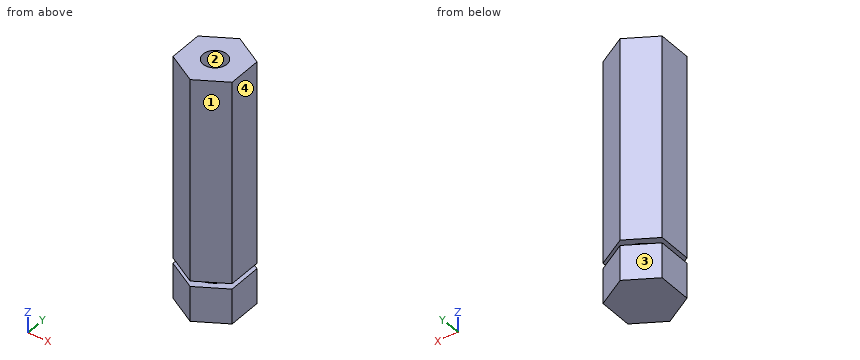
from build123d import *

# Parameters (mm, degrees)
BOSS_EXTRUDE1_DEPTH         = 26.19375
F_1_4_20_TAPPED_HOLE1_D     = 5.1054
F_1_4_20_TAPPED_HOLE1_DEPTH = 19.05
F_1_4_20_TAPPED_HOLE1_TIP   = 1.533816902
SKETCH5_W                   = 1.1684
SKETCH5_H                   = 4.843148419


with BuildPart() as part:
    # Sketch1 → Boss-Extrude1 (new body, symmetric)
    with BuildSketch(Plane.XY):
        Polygon((-6.35, 3.666174209), (-6.35, -3.666174209), (0, -7.332348419), (6.35, -3.666174209), (6.35, 3.666174209), (0, 7.332348419), align=None)
    extrude(amount=BOSS_EXTRUDE1_DEPTH, both=True)

    # 1/4-20 Tapped Hole1
    with Locations(Plane.XY.offset(26.19375)):
        with Locations((0, 0)):
            Hole(F_1_4_20_TAPPED_HOLE1_D / 2, depth=F_1_4_20_TAPPED_HOLE1_DEPTH)
            with Locations((0, 0, -(F_1_4_20_TAPPED_HOLE1_DEPTH + F_1_4_20_TAPPED_HOLE1_TIP / 2))):  # 118° drill point
                Cone(0, F_1_4_20_TAPPED_HOLE1_D / 2, F_1_4_20_TAPPED_HOLE1_TIP, mode=Mode.SUBTRACT)

    # Sketch5 → Cut-Revolve1 (revolve, cut)
    with BuildSketch(Plane(origin=(0, 0, 0), x_dir=(0, 0, -1), z_dir=(1, 0, 0))):
        with Locations((18.0467, 7.45077421)):
            Rectangle(SKETCH5_W, SKETCH5_H)
    revolve(axis=Axis((0, 0, -26.19375), (0, 0, 1)), mode=Mode.SUBTRACT)


solid = part.part
The model under review builds one solid part; all positions refer to its coordinate system, in mm. Face numbers are marked on the shaded views. Round coordinates to 2 decimals unless told otherwise and drop trailing zeros. Write each loop counter-clockwise with the first axis right and the second up, starting at its lowest first coordinate (ties: lowest second). Pieces come first, ordered by that corner, then holes. Notation, with made-up numbers: M -24.75,-12.75 L 14.25,-12.75 A23 ccw 14.25,0.25 Z; hole C -19.75,56 d11. An arc over 180 degrees is marked long. Use a Markdown table: item, result. Add a question column.
Q1. The part is to be moulded in two halves that separate along Y. For the marked faces 1, 2, 3 and 4, say which applies: pulls with the +Y half, pulls with the -Y half, needs draft (parallel to the pull), parting line crosses it, or undercut.
Q2. To check wall thickness, follow line 1 (Y direction, x = 0, z = 14); line 2 (X direction, y = 0, z = 18); line 3 (Z direction, x = -5, y = -2.5). State the ranges of each line that lie inside material, in increasing order.
Q3. Insertion check: pin 1 (1 mm diameter, centred on x = -1.5, y = 0.5, fed in from +Z); pin 2 (1 mm diameter, centred on x = -2.5, z = -10.5, fed in from -Y). Each pin has a flat end and moves straight along its axis. Give the tip position at first contact, or say it passes through.
Q4. We need section A-A, the plane z = 16. State the section outline as (x, y) points, plus the area to 3 significant figures.
Q5. We need section B-B, the plane z = -23. State the section outline as (x, y) points, plus the area to 3 significant figures.
Findings below:
| question | item | result |
|---|---|---|
| 1 | face 1 | pulls with the -Y half |
| 1 | face 2 | undercut |
| 1 | face 3 | pulls with the +Y half |
| 1 | face 4 | needs draft |
| 2 | line 1 | y = -7.33 to -2.55, 2.55 to 7.33 |
| 2 | line 2 | x = -6.35 to -2.55, 2.55 to 6.35 |
| 2 | line 3 | z = -26.19 to -18.63, -17.46 to 26.19 |
| 3 | pin 1 | stops at z = 6.86 |
| 3 | pin 2 | stops at y = -6.18 |
| 4 | outline | M -6.35,-3.67 L 0,-7.33 L 6.35,-3.67 L 6.35,3.67 L 0,7.33 L -6.35,3.67 Z; hole C 0,0 d5.11 |
| 4 | area | 119 mm² |
| 5 | outline | M -6.35,-3.67 L 0,-7.33 L 6.35,-3.67 L 6.35,3.67 L 0,7.33 L -6.35,3.67 Z |
| 5 | area | 140 mm² |
